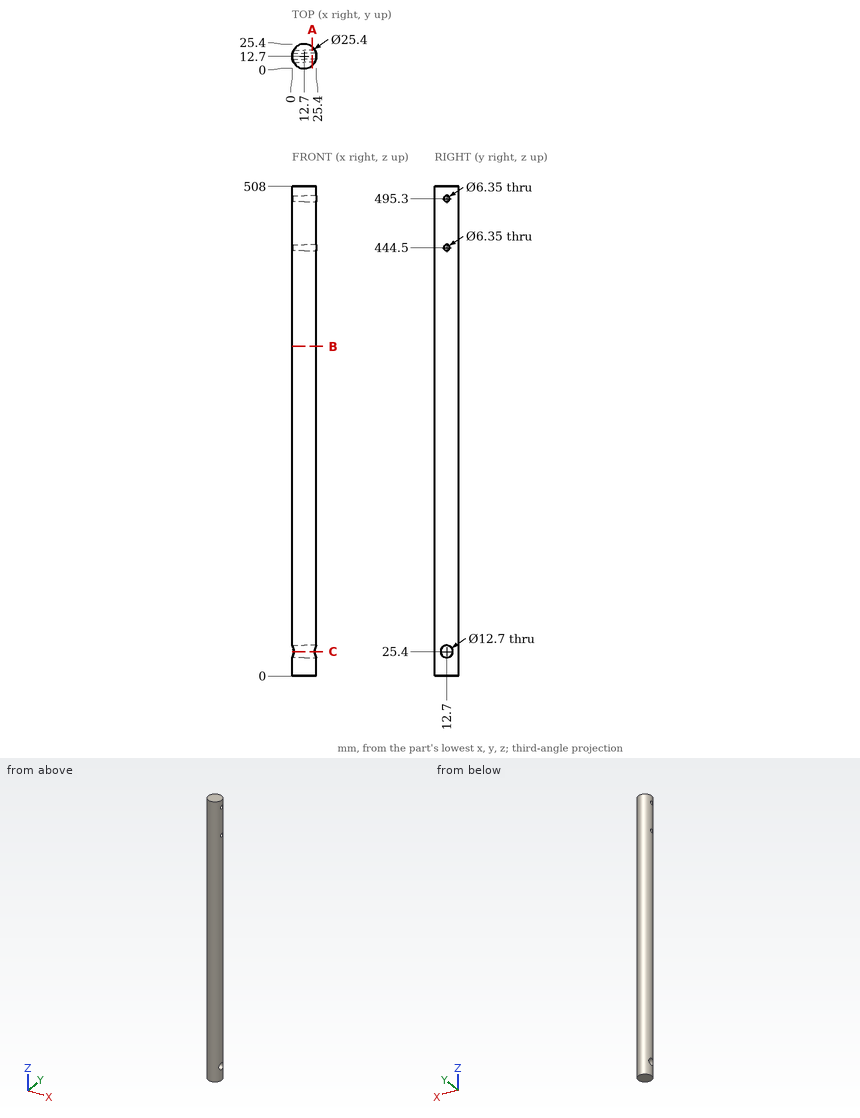
Answer from the drawing. Dimensions are ordinates in mm from the lowest x, y and z of the part. Round coordinates to 2 decimals unless told otherwise and drop trailing zeros. Loops run counter-clockwise (first coordinate to the right, second up) from the corner with the lowest first, then second, coordinate; pieces in that order, holes last.
Q1. Section A-A on x = 21 is taken. Give the number of separate pieces and of enclosed holes in the cut face, and give its area (3 significant figures).
Q2. Section C-C on z = 25.4 is taken. Write down the section's boundary in (x, y), and give its area (3 significant figures).
Q3. Each of these flat-tipped pins is pushed along its axis until it touches: pin 1 (3 mm diameter, centred on y = 9.5, z = 296.5, fed in from +X); pin 2 (2 mm diameter, centred on x = 11, z = 316, fed in from +Y); pin 3 (8 mm diameter, centred on y = 17.5, z = 218, fed in from -X). Where does it stop, or does it pass through?
Q4. Consider probe 1 along Z at (x, y) = (17, 13.25); probe 2 along Z at (x, y) = (1.75, 10); probe 3 along Z at (x, y) = (19.75, 17.5). Determine where each line is inside the solid, lowest interval first.
Q5. Section B-B on z = 342 is taken. Write down the section's boundary in (x, y).
Output:
1. separate pieces: 1
1. enclosed holes: 3
1. area: 9,580 mm2
2. outline: (1.7, 6.35) arc R12.7 ccw to (23.7, 6.35) - close; (1.7, 19.05) - (23.7, 19.05) arc R12.7 ccw to start
2. area: 198 mm2
3. pin 1: stops at x = 25.29
3. pin 2: stops at y = 25.38
3. pin 3: stops at x = 0.03
4. probe 1: z = 0 to 19.07, 31.73 to 441.37, 447.63 to 492.17, 498.43 to 508
4. probe 2: z = 0 to 19.65, 31.15 to 442.83, 446.17 to 493.63, 496.97 to 508
4. probe 3: z = 0 to 21.24, 29.56 to 508
5. outline: circle Ø25.4 at (12.7, 12.7)
